from build123d import *

# Parameters (mm, degrees)
SKETCH_1_W          = 86
SKETCH_1_H          = 26
SKETCH_1_W_2        = 9
SKETCH_1_H_2        = 2
EXTRUDE_1_DEPTH     = 1.5
SKETCH_3_W          = 86
SKETCH_3_H          = 3
EXTRUDE_2_DEPTH     = 6
SKETCH_4_R          = 2
CUT_EXTRUDE_1_DEPTH = 6


with BuildPart() as part:
    # 草图1 → 凸台-拉伸1 (new, symmetric)
    with BuildSketch(Plane.XY):
        with Locations((43, 13)):
            Rectangle(SKETCH_1_W, SKETCH_1_H)
        with Locations((14.5, 13)):
            Rectangle(SKETCH_1_W_2, SKETCH_1_H_2, mode=Mode.SUBTRACT)
        with Locations((33.5, 13)):
            Rectangle(SKETCH_1_W_2, SKETCH_1_H_2, mode=Mode.SUBTRACT)
        with Locations((52.5, 13)):
            Rectangle(SKETCH_1_W_2, SKETCH_1_H_2, mode=Mode.SUBTRACT)
        with Locations((71.5, 13)):
            Rectangle(SKETCH_1_W_2, SKETCH_1_H_2, mode=Mode.SUBTRACT)
    extrude(amount=EXTRUDE_1_DEPTH, both=True)

    # 草图3 → 凸台-拉伸2 (add)
    with BuildSketch(Plane(origin=(0, 0, -1.5), x_dir=(-1, 0, 0), z_dir=(0, 0, -1))):
        with Locations((-43, 1.5)):
            Rectangle(SKETCH_3_W, SKETCH_3_H)
    extrude(amount=EXTRUDE_2_DEPTH)

    # 草图4 → 切除-拉伸1 (cut)
    with BuildSketch(Plane(origin=(0, 3, 0), x_dir=(1, 0, 0), z_dir=(0, 1, 0))):
        with Locations(Location((10, 4.5, 0), (0, 0, 270))):
            Circle(SKETCH_4_R)
        with Locations(Location((76, 4.5, 0), (0, 0, 270))):
            Circle(SKETCH_4_R)
    extrude(amount=-CUT_EXTRUDE_1_DEPTH, mode=Mode.SUBTRACT)


solid = part.part
For this review, take the finished solid that the model builds, in its own axes (mm). A direction names the side the tool comes from. Coordinates: 2 decimals unless noted, no trailing zeros. Order: outer loops, then holes, each group sorted by start corner. A loop starts at its lowest first (then second) coordinate and runs counter-clockwise, first axis right, second up. Notation, with made-up numbers: (-18.5, 65.5) - (9.5, 65.5) arc R25 ccw to (9.5, 99.5) - close; hole circle Ø6 at (50, -26). An arc over 180 degrees is marked (long way). Answer as CSV lines item,"result". Start each with the question number.
1) Add section A-A (z = 0). State the section outline as (x, y) points, then the cut area to 3 significant figures.
2) Insertion check: P1, Ø5, axis at x = 54, z = -5.5, coming from the +Y side; P2, Ø1.5, axis at x = 53.5, z = 0.5, coming from the -Y side; P3, Ø1.5, axis at y = 14.5, z = -4, coming from the -X side. Each pin has a flat end and moves straight along its axis. Give the tip position at first contact, or say it passes through.
3) To check wall thickness, follow line 1 along X through (y, z) = (2.05, -4.5); line 2 along Y through (x, z) = (37, -0.25); line 3 along Y through (x, z) = (29, -2.75). State the ranges of each line that lie inside material, in increasing order. Write a range as [from, to].
4) Machinability: for faces 1 (the flat face through (42, 15, -1.5)), 2 (the cylindrical face through (11.352, 1.521, -5.974)), 3 (the flat face through (33, 14, 0)), which of the approach directions +Z, -Z, +X, -X, +Y, -Y give a long, thin tool a straight path to every point of the face, cutting with its end or side? Answer none if there is none.
5) Add section B-B (z = -4.5). State the section outline as (x, y) points.
6) Add section D-D (y = 5.25). State the section outline as (x, z) points, then the cut area to 3 significant figures.
7) Add section C-C (x = 27). State the section outline as (y, z) points.
8) Draft analysis for pull direction Z (two halves, no side actions). For faces 4 (the flat face through (44, 2, -7.5)), 5 (the flat face through (44, 0, -3)), 6 (the cylindrical face through (77.983, 1.521, -4.76)), state which applies: +Z half, -Z half, draft (parallel to the pull), parting line (faces both ways), or undercut.
Result:
1,outline,"(0, 0) - (86, 0) - (86, 26) - (0, 26) - close; hole (10, 12) - (19, 12) - (19, 14) - (10, 14) - close; hole (29, 12) - (38, 12) - (38, 14) - (29, 14) - close; hole (48, 12) - (57, 12) - (57, 14) - (48, 14) - close; hole (67, 12) - (76, 12) - (76, 14) - (67, 14) - close"
1,area,"2,160 mm^2"
2,P1,"y = 3"
2,P2,"y = 0"
2,P3,"through"
3,line 1,"[0, 8], [12, 74], [78, 86]"
3,line 2,"[0, 12], [14, 26]"
3,line 3,"[0, 3]"
4,face 1,"-Z, +X, -X, +Y"
4,face 2,"+Y, -Y"
4,face 3,"+Z, -Z"
5,outline,"(0, 0) - (8, 0) - (8, 3) - (0, 3) - close; (12, 0) - (74, 0) - (74, 3) - (12, 3) - close; (78, 0) - (86, 0) - (86, 3) - (78, 3) - close"
6,outline,"(0, -1.5) - (86, -1.5) - (86, 1.5) - (0, 1.5) - close"
6,area,"258 mm^2"
7,outline,"(0, -7.5) - (3, -7.5) - (3, -1.5) - (26, -1.5) - (26, 1.5) - (0, 1.5) - close"
8,face 4,"-Z half"
8,face 5,"draft"
8,face 6,"undercut"
